from build123d import *

# Parameters (mm, degrees)
SKETCH001_W   = 114
SKETCH001_H   = 5
SKETCH001_W_2 = 5
SKETCH001_H_2 = 154
PAD001_DEPTH  = 30
SKETCH_W      = 114
SKETCH_H      = 5
PAD_DEPTH     = 5
SKETCH002_W   = 114
SKETCH002_H   = 5
PAD002_DEPTH  = 18
SKETCH003_W   = 114
SKETCH003_H   = 5
PAD003_DEPTH  = 18


with BuildPart() as part:
    # Sketch001 → Pad001 (new body)
    with BuildSketch(Plane.XY):
        with Locations((57, 2.5)):
            Rectangle(SKETCH001_W, SKETCH001_H)
        with Locations((2.5, 82)):
            Rectangle(SKETCH001_W_2, SKETCH001_H_2)
        with Locations((111.5, 82)):
            Rectangle(SKETCH001_W_2, SKETCH001_H_2)
        with Locations((57, 161.5)):
            Rectangle(SKETCH001_W, SKETCH001_H)
    extrude(amount=PAD001_DEPTH)

    # Sketch → Pad (new body)
    with BuildSketch(Plane.XY.offset(30)):
        with Locations((57, 161.5)):
            Rectangle(SKETCH_W, SKETCH_H)
        with Locations((57, 2.5)):
            Rectangle(SKETCH_W, SKETCH_H)
    extrude(amount=PAD_DEPTH)

    # Sketch002 → Pad002 (new body)
    with BuildSketch(Plane.XZ):
        with Locations((57, 32.5)):
            Rectangle(SKETCH002_W, SKETCH002_H)
    extrude(amount=PAD002_DEPTH)

    # Sketch003 → Pad003 (new body)
    with BuildSketch(Plane(origin=(0, 164, 0), x_dir=(-1, 0, 0), z_dir=(0, 1, 0))):
        with Locations((-57, 32.5)):
            Rectangle(SKETCH003_W, SKETCH003_H)
    extrude(amount=PAD003_DEPTH)


solid = part.part
The listing builds one solid part. Answer for the finished solid, in the listing's coordinates (mm). A direction names the side the tool comes from. Give positions to 0.01 mm unless a question says otherwise; leave off trailing zeros. Write each loop counter-clockwise with the first axis right and the second up, starting at its lowest first coordinate (ties: lowest second). Pieces come first, ordered by that corner, then holes. Notation, with made-up numbers: (23.5, 54) - (69.5, 54) arc R26 cw to (69.5, 78) - close; hole circle Ø9 at (-13, 48). An arc over 180 degrees is marked (long way). Use a Markdown table: item, result.
1. Each of these flat-tipped pins is pushed along its axis until it touches: P1, Ø1, axis at x = 16, z = 23.5, coming from the -Y side; P2, Ø2, axis at x = 69.5, z = 12, coming from the +Y side; P3, Ø2.5, axis at x = 3, y = 116, coming from the +Z side. Where does it stop, or does it pass through?
Values follow:
| item | result |
|---|---|
| P1 | stops at y = 0 |
| P2 | stops at y = 164 |
| P3 | stops at z = 30 |
2. Find the intervals of material crossed by probe 1 along X at (y, z) = (123, 20.5); probe 2 along Y at (x, z) = (75.5, 25); probe 3 along Z at (x, y) = (109.5, 64.5), in increasing order. Write a range as from..to.
Values follow:
| item | result |
|---|---|
| probe 1 | x = 0..5, 109..114 |
| probe 2 | y = 0..5, 159..164 |
| probe 3 | z = 0..30 |
3. A tool of negligible diameter and unlimited length cuts with its end or side. For faces 1 (the flat face through (2, 83, 30)), 2 (the flat face through (109, 81, 15)), 3 (the flat face through (56, -9, 30)), 4 (the flat face through (58, 173, 30)), from which of +Z, -Z, +X, -X, +Y, -Y can it reach the whole face along a straight path? Write none if from no direction.
Values follow:
| item | result |
|---|---|
| face 1 | +Z, +X, -X |
| face 2 | +Z, -Z |
| face 3 | -Z, +X, -X, -Y |
| face 4 | -Z, +X, -X, +Y |
4. Section C-C on y = 107.5 is taken. Write down the section's boundary in (x, z), plus the area to 3 significant figures.
Values follow:
| item | result |
|---|---|
| outline | (0, 0) - (5, 0) - (5, 30) - (0, 30) - close; (109, 0) - (114, 0) - (114, 30) - (109, 30) - close |
| area | 300 mm² |
5. Section A-A on z = 28 is taken. Write down the section's boundary in (x, y).
Values follow:
| item | result |
|---|---|
| outline | (0, 0) - (114, 0) - (114, 164) - (0, 164) - close; hole (5, 5) - (109, 5) - (109, 159) - (5, 159) - close |
6. Section B-B on x = 56.5 is taken. Write down the section's boundary in (y, z), plus the area to 3 significant figures.
Values follow:
| item | result |
|---|---|
| outline | (-18, 30) - (0, 30) - (0, 0) - (5, 0) - (5, 35) - (-18, 35) - close; (159, 0) - (164, 0) - (164, 30) - (182, 30) - (182, 35) - (159, 35) - close |
| area | 530 mm² |
7. For a pull along X with two mould halves and no side action, classify faces 5 (the flat face through (0, 81, 17)), 6 (the flat face through (5, 81, 15)), 7 (the flat face through (56, 5, 17)), 8 (the flat face through (56, 0, 15)) as released by +X, released by -X, zero draft, split by the parting line, or undercut.
Values follow:
| item | result |
|---|---|
| face 5 | released by -X |
| face 6 | undercut |
| face 7 | undercut |
| face 8 | zero draft |
